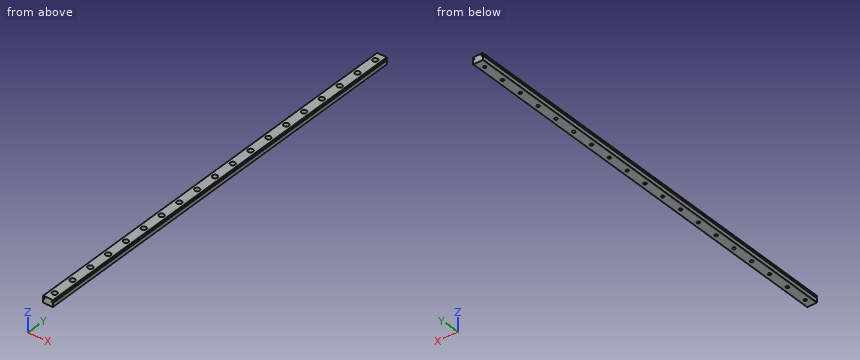
```python
from build123d import *

# Parameters (mm, degrees)
PAD_DEPTH           = 500
SKETCH001_R         = 3
POCKET_DEPTH        = 4.5
SKETCH002_R         = 1.75
POCKET001_DEPTH     = 8.001
LINEARPATTERN_COUNT = 19
LINEARPATTERN_PITCH = 26.666667


with BuildPart() as part:
    # Sketch → Pad (new body)
    with BuildSketch(Plane.XZ):
        with BuildLine():
            Line((-5.5, 0), (5.5, 0))
            ThreePointArc((5.5, 0), (5.853553, 0.146447), (6, 0.5))
            Line((6, 0.5), (6, 4.5))
            ThreePointArc((6, 4.5), (5.853553, 4.853553), (5.5, 5))
            Line((5.5, 5), (4, 5))
            Line((4, 5), (4, 6))
            Line((4, 6), (5.5, 6))
            ThreePointArc((5.5, 6), (5.853553, 6.146447), (6, 6.5))
            Line((6, 6.5), (6, 7.5))
            ThreePointArc((6, 7.5), (5.853553, 7.853553), (5.5, 8))
            Line((-5.5, 8), (5.5, 8))
            ThreePointArc((-5.5, 8), (-5.853553, 7.853553), (-6, 7.5))
            Line((-6, 6.5), (-6, 7.5))
            ThreePointArc((-6, 6.5), (-5.853553, 6.146447), (-5.5, 6))
            Line((-4, 6), (-5.5, 6))
            Line((-4, 5), (-4, 6))
            Line((-5.5, 5), (-4, 5))
            ThreePointArc((-5.5, 5), (-5.853553, 4.853553), (-6, 4.5))
            Line((-6, 0.5), (-6, 4.5))
            ThreePointArc((-6, 0.5), (-5.853553, 0.146447), (-5.5, 0))
        make_face()
    extrude(amount=PAD_DEPTH)

    # Sketch001 (on Face12 of Pad) → Pocket (cut)
    with BuildSketch(Plane(origin=(0, 0, 8), x_dir=(-1, 0, 0), z_dir=(0, 0, 1))):
        with Locations((0, 10)):
            Circle(SKETCH001_R)
    pocket = extrude(amount=-POCKET_DEPTH, mode=Mode.SUBTRACT)

    # Sketch002 (on Face16 of Pocket) → Pocket001 (cut, through all)
    with BuildSketch(Plane(origin=(0, 0, 8), x_dir=(-1, 0, 0), z_dir=(0, 0, 1))):
        with Locations((0, 10)):
            Circle(SKETCH002_R)
    pocket001 = extrude(amount=-POCKET001_DEPTH, mode=Mode.SUBTRACT)

    # LinearPattern: Pocket, Pocket001 ×19
    with Locations(*[(0, -i * LINEARPATTERN_PITCH, 0) for i in range(1, LINEARPATTERN_COUNT)]):
        add(pocket, mode=Mode.SUBTRACT)
        add(pocket001, mode=Mode.SUBTRACT)


solid = part.part
```
Could you check a few things on this model? Use its own coordinates, in mm. Coordinates: 2 decimals unless noted, no trailing zeros. Write each loop counter-clockwise with the first axis right and the second up, starting at its lowest first coordinate (ties: lowest second). Pieces come first, ordered by that corner, then holes. Notation, with made-up numbers: (21.25, 14.5) -> (43.25, 14.5) arc R22 cw to (43.25, 30.5) -> close; hole circle Ø1 at (24, 83.25). An arc over 180 degrees is marked (long way). Write item = value, one per line. Start each with the question number.
(1) Will these pins go through, and if not, where does the flat tip stop? pin 1 (2 mm diameter, centred on x = 0, y = -143.33, fed in from -Z); pin 2 (6 mm diameter, centred on x = 1.5, y = -191.5, fed in from -Z); pin 3 (4 mm diameter, centred on x = 0, y = -170, fed in from +Z).
(2) I want a section at A-A (y = -212.5). Please give me the cut outline in (x, z), plus the area to 3 significant figures.
(3) I want a section at B-B (z = 2). Give the number of separate pieces and of enclosed holes in the cut face, plus the area to 3 significant figures.
(4) I need wall thicknesses on line 1 (Z direction, x = 5, y = -105); line 2 (Z direction, x = 5.75, y = -75.5); line 3 (X direction, y = -180, z = 5.25). Which ranges of each line are inside material? Lowest first, please. Write a range as [from, to].
Result set:
q1.pin_1 = through
q1.pin_2 = 0
q1.pin_3 = 3.5
q2.outline = (-6, 0.5) arc R0.5 ccw to (-5.5, 0) -> (5.5, 0) arc R0.5 ccw to (6, 0.5) -> (6, 4.5) arc R0.5 ccw to (5.5, 5) -> (4, 5) -> (4, 6) -> (5.5, 6) arc R0.5 ccw to (6, 6.5) -> (6, 7.5) arc R0.5 ccw to (5.5, 8) -> (-5.5, 8) arc R0.5 ccw to (-6, 7.5) -> (-6, 6.5) arc R0.5 ccw to (-5.5, 6) -> (-4, 6) -> (-4, 5) -> (-5.5, 5) arc R0.5 ccw to (-6, 4.5) -> close
q2.area = 91.6 mm2
q3.separate_pieces = 1
q3.enclosed_holes = 19
q3.area = 5,820 mm2
q4.line_1 = [0, 5], [6, 8]
q4.line_2 = [0.07, 4.93], [6.07, 7.93]
q4.line_3 = [-4, 4]
